```python
from build123d import *

# Parameters (mm, degrees)
F0_W          = 75.946
F0_H          = 152.4
F2_DEPTH      = 6.35
F1_W          = 6.35
F1_H          = 152.4
F3_DEPTH      = 35
F4_R          = 2.54
F5_DEPTH      = 41.351
F7_DEPTH      = 6.351
F7_DEPTH_BACK = 69.597


with BuildPart() as f2:
    # F0 (on Top) → F2 (new body)
    with BuildSketch(Plane.XY):
        with Locations((37.973, 76.2)):
            Rectangle(F0_W, F0_H)
    extrude(amount=-F2_DEPTH)

    # F1 (on face) → F3 (join)
    with BuildSketch(Plane.XY):
        with Locations((3.175, 76.2)):
            Rectangle(F1_W, F1_H)
        with Locations((72.517, 76.2)):
            Rectangle(F1_W, F1_H)
    extrude(amount=F3_DEPTH)

    # F4 (on face) → F5 (cut, through all)
    with BuildSketch(Plane(origin=(0, 0, -6.35), x_dir=(1, 0, 0), z_dir=(0, 0, -1))):
        with Locations((57.15, -12.7)):
            Circle(F4_R)
        with Locations((19.05, -12.7)):
            Circle(F4_R)
        with Locations((19.05, -139.7)):
            Circle(F4_R)
        with Locations((57.15, -139.7)):
            Circle(F4_R)
    extrude(amount=-F5_DEPTH, mode=Mode.SUBTRACT)

    # F6 (on face) → F7 (cut, two sides)
    with BuildSketch(Plane.YZ.offset(6.35)) as f7_sk:
        with BuildLine():
            ThreePointArc((31.75, 12.192), (27.4139487758, 13.9880512242), (29.21, 9.652))
            Line((29.21, 9.652), (29.21, 12.192))
            Line((29.21, 12.192), (31.75, 12.192))
        make_face()
        with BuildLine():
            ThreePointArc((125.73, 12.192), (123.19, 14.732), (120.65, 12.192))
            Line((120.65, 12.192), (123.19, 12.192))
            Line((123.19, 12.192), (123.19, 9.652))
            ThreePointArc((123.19, 9.652), (124.9860512242, 10.3959487758), (125.73, 12.192))
        make_face()
        with BuildLine():
            Line((123.19, 12.192), (120.65, 12.192))
            ThreePointArc((120.65, 12.192), (121.3939487758, 10.3959487758), (123.19, 9.652))
            Line((123.19, 9.652), (123.19, 12.192))
        make_face()
        with BuildLine():
            Line((29.21, 12.192), (29.21, 9.652))
            ThreePointArc((29.21, 9.652), (31.0060512242, 10.3959487758), (31.75, 12.192))
            Line((31.75, 12.192), (29.21, 12.192))
        make_face()
    extrude(amount=-F7_DEPTH, mode=Mode.SUBTRACT)
    extrude(f7_sk.sketch, amount=F7_DEPTH_BACK, mode=Mode.SUBTRACT)


solid = f2.part
```
Geometry check sheet. Reference: the model listing, model coordinates, mm. A direction names the side the tool comes from. Coordinates: 2 decimals unless noted, no trailing zeros. Order: outer loops, then holes, each group sorted by start corner. A loop starts at its lowest first (then second) coordinate and runs counter-clockwise, first axis right, second up.
Q1. Sectioned sample at A-A on y = 139.7. Record the cut outline in (x, z).
Reply:
outline: (0, -6.35) - (16.51, -6.35) - (16.51, 0) - (6.35, 0) - (6.35, 35) - (0, 35) - close; (21.59, -6.35) - (54.61, -6.35) - (54.61, 0) - (21.59, 0) - close; (59.69, -6.35) - (75.95, -6.35) - (75.95, 0) - (75.69, 0) - (75.69, 35) - (69.34, 35) - (69.34, 0) - (59.69, 0) - close
Q2. Draft check along Y on faces 4 (the face through (75.946, 75, -3)), 5 (the face through (38, 152.4, -1)), 6 (the face through (54.612, 139.588, -3.219)). Enter one of: released by +Y, released by -Y, zero draft, split by the parting line, or undercut.
Reply:
face 4: zero draft
face 5: released by +Y
face 6: undercut
Q3. Tool access check on faces 1 (the face through (75.692, 75, 17)), 2 (the face through (0, 75, 14)), 3 (the face through (37, 77, 0)). Record the directions out of +Z, -Z, +X, -X, +Y, -Y that give a thin tool (end or side, any length) a straight path to the whole face; none if there is none.
Reply:
face 1: +Z, +X, +Y, -Y
face 2: +Z, -Z, -X, +Y, -Y
face 3: +Z, +Y, -Y
Q4. Thickness scan on probe 1 along Y at (x, z) = (19.05, -1.75); probe 2 along Z at (x, y) = (2, 29); probe 3 along X at (y, z) = (131.5, 27.5). Record the ranges inside material, lowest first.
Reply:
probe 1: y = 0 to 10.16, 15.24 to 137.16, 142.24 to 152.4
probe 2: z = -6.35 to 9.66, 14.72 to 35
probe 3: x = 0 to 6.35, 69.34 to 75.69
Q5. Sectioned sample at B-B on x = 19.05. Record the cut outline in (y, z).
Reply:
outline: (0, -6.35) - (10.16, -6.35) - (10.16, 0) - (0, 0) - close; (15.24, -6.35) - (137.16, -6.35) - (137.16, 0) - (15.24, 0) - close; (142.24, -6.35) - (152.4, -6.35) - (152.4, 0) - (142.24, 0) - close
Q6. Sectioned sample at C-C on z = 31.5. Record the cut outline in (x, y), and give its area (3 significant figures).
Reply:
outline: (0, 0) - (6.35, 0) - (6.35, 152.4) - (0, 152.4) - close; (69.34, 0) - (75.69, 0) - (75.69, 152.4) - (69.34, 152.4) - close
area: 1,940 mm2
Q7. Depth check by flat-ended pin: pin 1 Ø8 at (x, y) = (19.05, 139.7) entering from +Z; pin 2 Ø10.5 at (y, z) = (105.5, 13.5) entering from -X. Enter the tip coordinate at first touch or a pass-through.
Reply:
pin 1: stops at z = 0
pin 2: stops at x = 0
Q8. Sectioned sample at D-D on y = 23.5. Record the cut outline in (x, z).
Reply:
outline: (0, -6.35) - (75.95, -6.35) - (75.95, 0) - (75.69, 0) - (75.69, 35) - (69.34, 35) - (69.34, 0) - (6.35, 0) - (6.35, 35) - (0, 35) - close
